Can you work these out from the model? Positions are in its coordinate system, mm. A direction names the side the tool comes from. Coordinates: 2 decimals unless noted, no trailing zeros. Order: outer loops, then holes, each group sorted by start corner. A loop starts at its lowest first (then second) coordinate and runs counter-clockwise, first axis right, second up. Notation, with made-up numbers: (-32.75, 41) -> (1.25, 41) arc R22 cw to (1.25, 71) -> close; hole circle Ø1 at (42.25, -24.75). An arc over 180 degrees is marked (long way). Use a Markdown table: item, result. Add a question column.
1. Suppose I cut it at A-A, the plane z = 0. State how many separate pieces and enclosed holes the cut face has, then the cut area to 3 significant figures.
2. We'd pull the mould along Z, two halves only. Please class faces 5 (the flat face through (-7, 4, 21)), 6 (the flat face through (0, 3, -39.8)), 7 (the flat face through (0, 1, -28)), 8 (the flat face through (0, 12, -4.5)): pulls with the +Z half, pulls with the -Z half, needs draft (parallel to the pull), parting line crosses it, or undercut.
3. If I drill on line 1 along Z through (x, y) = (-7, 3.3); line 2 along X through (y, z) = (3.3, -21.6); line 3 along X through (y, z) = (11.05, 28.8), over which ranges is the centre line in solid material (lowest first)? Write a range as from..to.
4. Suppose I cut it at B-B, the plane y = 5. List the corners of the cut face in (x, z) for me.
5. Suppose I cut it at D-D, the plane y = 27.9. List the corners of the cut face in (x, z) for me, then the cut area to 3 significant figures.
6. For pin 1 Ø7 at (y, z) = (2.5, 27) entering from +X; pin 2 Ø1.2 at (x, y) = (-19.5, 43) entering from -Z; pin 3 Ø3.5 at (x, z) = (-13, 13) entering from -Y; pin 4 Ø8 at (y, z) = (48, 18.5) entering from -X, each with a flat end and sliding along its axis, tell me the tip position at first contact or that it passes through.
7. For faces 1 (the cylindrical face through (-12.01, 1.97, -11.09)), 2 (the flat face through (-19, 43, -8)), 3 (the flat face through (-14, 54.1, 0)), 4 (the flat face through (6.25, 11, -9)), which set-ups out of +Z, -Z, +X, -X, +Y, -Y let a thin tool reach every point of the face, with its end or its side?
8. Suppose I cut it at C-C, the plane z = 13. List the corners of the cut face in (x, y) for me.
```python
from build123d import *

# Parameters (mm, degrees)
SKETCH_1_W                 = 62.3
SKETCH_1_H                 = 34
EXTRUDE_346_DEPTH          = 4
HOLE_WIZARD_M4_1_D         = 4.3
PATTERN_SKETCH_1_OUTLINE_R = 2.15
PATTERN_SKETCH_1_DEPTH     = 4
SKETCH_6_W                 = 22.72
SKETCH_6_H                 = 3
EXTRUDE_2_DEPTH            = 22.8
HOLE_WIZARD_M2_5_1_D       = 2.7
PATTERN_START              = 1
PATTERN_SKETCH_2_OUTLINE_R = 1.35
PATTERN_SKETCH_2_DEPTH     = 3
SKETCH_11_W                = 25.6
SKETCH_11_H                = 4
EXTRUDE_5_DEPTH            = 4
SKETCH_12_W                = 25.6
SKETCH_12_H                = 4
EXTRUDE_6_DEPTH            = 9
SKETCH_13_W                = 25.6
SKETCH_13_H                = 4
EXTRUDE_7_DEPTH            = 16.8
HOLE_WIZARD_M2_1_D         = 2.2
EXTRUDE_START              = -14
EXTRUDE_8_OUTLINE_W        = 12.5
EXTRUDE_8_OUTLINE_H        = 20.251
EXTRUDE_8_OUTLINE_R        = 0.25
EXTRUDE_8_DEPTH            = 9.5
CUT_EXTRUDE_1_REACH        = 67.128
SKETCH_18_R                = 3.2
FILLET_1_RADIUS            = 6.25
FILLET_1_LENGTH            = 9.5
SKETCH_19_W                = 4
SKETCH_19_H                = 24
EXTRUDE_10_DEPTH           = 29
SKETCH_20_W                = 8
SKETCH_20_H                = 1
EXTRUDE_11_DEPTH           = 22.15
CUT_EXTRUDE_3_REACH        = 62.36
SKETCH_22_W                = 1.6
SKETCH_22_H                = 3
FILLET_2_RADIUS            = 0.5
FILLET_2_LENGTH            = 3
FILLET_3_R                 = 0.5
SKETCH_23_W                = 1
SKETCH_23_H                = 9
EXTRUDE_12_DEPTH           = 16.8
HOLE_WIZARD_M3_1_D         = 3.2
EXTRUDE_START_2            = 29
SKETCH_19_2_W              = 4
SKETCH_19_2_H              = 24
EXTRUDE_17_DEPTH           = 29.1
CUT_EXTRUDE_4_REACH        = 90.167
SKETCH_29_W                = 16
SKETCH_29_H                = 21.1
SKETCH_30_W                = 24
SKETCH_30_H                = 8
EXTRUDE_18_DEPTH           = 13.25
CHAMFER_1_SIZE             = 3
FILLET_4_R                 = 2.414214


# Read off the part's stored shape, not the designer's step: 草图阵列1, 草图阵列2, 凸台-拉伸8
with BuildPart() as part:
    # 草图1 → Extrude 346 (new body)
    with BuildSketch(Plane(origin=(0, 0, 0), x_dir=(1, 0, 0), z_dir=(0, 1, 0))):
        Rectangle(SKETCH_1_W, SKETCH_1_H)
    extrude(amount=EXTRUDE_346_DEPTH)

    # M4 间隙孔1 (through all)
    with Locations(Plane(origin=(0, 4, 0), x_dir=(1, 0, 0), z_dir=(0, 1, 0))):
        with Locations((13, -13)):
            Hole(HOLE_WIZARD_M4_1_D / 2)

    # 草图阵列1 outline → 草图阵列1 (cut)
    with BuildSketch(Plane(origin=(0, 0, 0), x_dir=(1, 0, 0), z_dir=(0, 1, 0))):
        with Locations((-13, 13)):
            Circle(PATTERN_SKETCH_1_OUTLINE_R)
        with Locations((-13, -13)):
            Circle(PATTERN_SKETCH_1_OUTLINE_R)
        with Locations((13, 13)):
            Circle(PATTERN_SKETCH_1_OUTLINE_R)
    extrude(amount=PATTERN_SKETCH_1_DEPTH, mode=Mode.SUBTRACT)

    # 草图6 → 凸台-拉伸2 (add)
    with BuildSketch(Plane(origin=(0, 0, -17), x_dir=(-1, 0, 0), z_dir=(0, 0, -1))):
        with Locations((0, 2.5)):
            Rectangle(SKETCH_6_W, SKETCH_6_H)
    extrude(amount=EXTRUDE_2_DEPTH)

    # M2.5 间隙孔1 (through all)
    with Locations(Plane(origin=(0, 4, 0), x_dir=(1, 0, 0), z_dir=(0, 1, 0))):
        with Locations((-7, 35.6)):
            Hole(HOLE_WIZARD_M2_5_1_D / 2)

    # 草图阵列2 outline → 草图阵列2 (cut)
    with BuildSketch(Plane(origin=(0, 0, 0), x_dir=(1, 0, 0), z_dir=(0, 1, 0)).offset(PATTERN_START)):
        with Locations((7, 21.6)):
            Circle(PATTERN_SKETCH_2_OUTLINE_R)
        with Locations((7, 35.6)):
            Circle(PATTERN_SKETCH_2_OUTLINE_R)
        with Locations((-7, 21.6)):
            Circle(PATTERN_SKETCH_2_OUTLINE_R)
    extrude(amount=PATTERN_SKETCH_2_DEPTH, mode=Mode.SUBTRACT)

    # 草图11 → 凸台-拉伸5 (add)
    with BuildSketch(Plane.XY.offset(17)):
        with Locations((0, 2)):
            Rectangle(SKETCH_11_W, SKETCH_11_H)
    extrude(amount=EXTRUDE_5_DEPTH)

    # 草图12 → 凸台-拉伸6 (add)
    with BuildSketch(Plane(origin=(0, 4, 0), x_dir=(1, 0, 0), z_dir=(0, 1, 0))):
        with Locations((0, -19)):
            Rectangle(SKETCH_12_W, SKETCH_12_H)
    extrude(amount=EXTRUDE_6_DEPTH)

    # 草图13 → 凸台-拉伸7 (add)
    with BuildSketch(Plane.XY.offset(21)):
        with Locations((0, 11)):
            Rectangle(SKETCH_13_W, SKETCH_13_H)
    extrude(amount=EXTRUDE_7_DEPTH)

    # M2 间隙孔1 (through all)
    with Locations(Plane(origin=(0, 9, 0), x_dir=(-1, 0, 0), z_dir=(0, -1, 0))):
        with Locations((8.9, -28.8), (-8.9, -28.8)):
            Hole(HOLE_WIZARD_M2_1_D / 2)

    # 凸台-拉伸8 outline → 凸台-拉伸8 (add)
    with BuildSketch(Plane.XY.offset(EXTRUDE_START)):
        with Locations((0, 14.1255)):
            Rectangle(EXTRUDE_8_OUTLINE_W, EXTRUDE_8_OUTLINE_H)
        with Locations((0, 18)):
            Circle(EXTRUDE_8_OUTLINE_R, mode=Mode.SUBTRACT)
    extrude(amount=EXTRUDE_8_DEPTH)

    # 草图18 → 切除-拉伸1 (cut, up to next)
    with BuildSketch(Plane(origin=(0, 0, -14), x_dir=(-1, 0, 0), z_dir=(0, 0, -1)), mode=Mode.PRIVATE) as cut_extrude_1_sk1:
        with Locations((0, 18)):
            Circle(SKETCH_18_R)
    cut_extrude_1_tool1 = extrude(cut_extrude_1_sk1.sketch, amount=-CUT_EXTRUDE_1_REACH, mode=Mode.PRIVATE) & part.part
    add(cut_extrude_1_tool1.solids().sort_by_distance((0, 18, -14))[0], mode=Mode.SUBTRACT)

    # 圆角1: full round fillet: the end face becomes a half cylinder, R = half its width
    fillet_1_face = Plane((0, 24.251, -9.25), x_dir=(0, 0, -1), z_dir=(0, 1, 0))  # on the end face: x along it, z out of the body
    fillet_1_slab = fillet_1_face.offset(-FILLET_1_RADIUS / 2) * Box(FILLET_1_LENGTH, 2 * FILLET_1_RADIUS, FILLET_1_RADIUS, mode=Mode.PRIVATE)  # the body's end, R deep
    fillet_1_round = Plane((0, 18.001, -9.25), x_dir=(0, 1, 0), z_dir=(0, 0, -1)) * Cylinder(FILLET_1_RADIUS, FILLET_1_LENGTH, mode=Mode.PRIVATE)  # its axis R under the face
    add(fillet_1_slab - fillet_1_round, mode=Mode.SUBTRACT)

    # 草图19 → 凸台-拉伸10 (add)
    with BuildSketch(Plane(origin=(0, 4, 0), x_dir=(1, 0, 0), z_dir=(0, 1, 0))):
        with Locations((-19.15, 0)):
            Rectangle(SKETCH_19_W, SKETCH_19_H)
    extrude(amount=EXTRUDE_10_DEPTH)

    # 草图20 → 凸台-拉伸11 (add)
    with BuildSketch(Plane(origin=(-17.15, 0, 0), x_dir=(0, 0, -1), z_dir=(1, 0, 0))):
        with Locations((0, 32.5)):
            Rectangle(SKETCH_20_W, SKETCH_20_H)
    extrude(amount=EXTRUDE_11_DEPTH)

    # 草图22 → 切除-拉伸3 (cut, up to next)
    with BuildSketch(Plane(origin=(0, 33, 0), x_dir=(1, 0, 0), z_dir=(0, 1, 0)), mode=Mode.PRIVATE) as cut_extrude_3_sk1:
        Rectangle(SKETCH_22_W, SKETCH_22_H)
    cut_extrude_3_tool1 = extrude(cut_extrude_3_sk1.sketch, amount=-CUT_EXTRUDE_3_REACH, mode=Mode.PRIVATE) & part.part
    add(cut_extrude_3_tool1.solids().sort_by_distance((0, 33, 0))[0], mode=Mode.SUBTRACT)

    # 圆角2: full round fillet: the end face becomes a half cylinder, R = half its width
    fillet_2_face = Plane((-0.8, 32.5, 0), x_dir=(0, 0, -1), z_dir=(1, 0, 0))  # on the end face: x along it, z out of the body
    fillet_2_slab = fillet_2_face.offset(-FILLET_2_RADIUS / 2) * Box(FILLET_2_LENGTH, 2 * FILLET_2_RADIUS, FILLET_2_RADIUS, mode=Mode.PRIVATE)  # the body's end, R deep
    fillet_2_round = Plane((-1.3, 32.5, 0), x_dir=(1, 0, 0), z_dir=(0, 0, -1)) * Cylinder(FILLET_2_RADIUS, FILLET_2_LENGTH, mode=Mode.PRIVATE)  # its axis R under the face
    add(fillet_2_slab - fillet_2_round, mode=Mode.SUBTRACT)

    # 圆角3
    fillet_3_edges = [part.edges().sort_by_distance(p)[0] for p in [
        (0.8, 33, 0),
    ]]
    fillet(fillet_3_edges, radius=FILLET_3_R)

    # 草图23 → 凸台-拉伸12 (add)
    with BuildSketch(Plane.XY.offset(21)):
        with Locations((0, 4.5)):
            Rectangle(SKETCH_23_W, SKETCH_23_H)
    extrude(amount=EXTRUDE_12_DEPTH)

    # M3 间隙孔1 (through all)
    with Locations(Plane(origin=(-17.15, 0, 0), x_dir=(0, 0, -1), z_dir=(1, 0, 0))):
        with Locations((0, 27.9)):
            Hole(HOLE_WIZARD_M3_1_D / 2)

    # 草图19<2> → 凸台-拉伸17 (add)
    with BuildSketch(Plane(origin=(0, 4, 0), x_dir=(1, 0, 0), z_dir=(0, 1, 0)).offset(EXTRUDE_START_2)):
        with Locations((-19.15, 0)):
            Rectangle(SKETCH_19_2_W, SKETCH_19_2_H)
    extrude(amount=EXTRUDE_17_DEPTH)

    # 草图29 → 切除-拉伸4 (cut, up to next)
    with BuildSketch(Plane(origin=(-17.15, 0, 0), x_dir=(0, 0, -1), z_dir=(1, 0, 0)), mode=Mode.PRIVATE) as cut_extrude_4_sk1:
        with Locations((0, 43.55)):
            Rectangle(SKETCH_29_W, SKETCH_29_H)
    cut_extrude_4_tool1 = extrude(cut_extrude_4_sk1.sketch, amount=-CUT_EXTRUDE_4_REACH, mode=Mode.PRIVATE) & part.part
    add(cut_extrude_4_tool1.solids().sort_by_distance((-17.15, 43.55, 0))[0], mode=Mode.SUBTRACT)

    # 草图30 → 凸台-拉伸18 (add)
    with BuildSketch(Plane(origin=(-17.15, 0, 0), x_dir=(0, 0, -1), z_dir=(1, 0, 0))):
        with Locations((0, 58.1)):
            Rectangle(SKETCH_30_W, SKETCH_30_H)
    extrude(amount=EXTRUDE_18_DEPTH)

    # 倒角1
    chamfer_1_edges = [part.edges().sort_by_distance(p)[0] for p in [
        (-3.9, 62.1, 0),
        (-3.9, 54.1, 0),
    ]]
    chamfer(chamfer_1_edges, length=CHAMFER_1_SIZE)

    # 圆角4
    fillet_4_edges = [part.edges().sort_by_distance(p)[0] for p in [
        (-3.9, 57.1, 0),
        (-3.9, 59.1, 0),
    ]]
    fillet(fillet_4_edges, radius=FILLET_4_R - 0.0001)  # a hair under: the kernel refuses the full size


solid = part.part
```
Worked out:
| question | item | result |
|---|---|---|
| 1 | separate pieces | 4 |
| 1 | enclosed holes | 0 |
| 1 | area | 502 mm² |
| 2 | face 5 | pulls with the +Z half |
| 2 | face 6 | pulls with the -Z half |
| 2 | face 7 | needs draft |
| 2 | face 8 | undercut |
| 3 | line 1 | z = -39.8..-36.95, -34.25..-22.95, -20.25..21 |
| 3 | line 2 | x = -11.36..-8.35, -5.65..5.65, 8.35..11.36 |
| 3 | line 3 | x = -12.8..-10, -7.8..7.8, 10..12.8 |
| 4 | outline | (-21.15, -12) -> (-17.15, -12) -> (-17.15, 12) -> (-21.15, 12) -> close; (-12.8, 17) -> (12.8, 17) -> (12.8, 21) -> (0.5, 21) -> (0.5, 37.8) -> (-0.5, 37.8) -> (-0.5, 21) -> (-12.8, 21) -> close; (-6.25, -14) -> (6.25, -14) -> (6.25, -4.5) -> (-6.25, -4.5) -> close |
| 5 | outline | (-21.15, -12) -> (-17.15, -12) -> (-17.15, -1.6) -> (-21.15, -1.6) -> close; (-21.15, 1.6) -> (-17.15, 1.6) -> (-17.15, 12) -> (-21.15, 12) -> close |
| 5 | area | 83.2 mm² |
| 6 | pin 1 | stops at x = 0.5 |
| 6 | pin 2 | stops at z = -12 |
| 6 | pin 3 | stops at y = 54.1 |
| 6 | pin 4 | passes through |
| 7 | face 1 | -Y |
| 7 | face 2 | +X, -X |
| 7 | face 3 | +X |
| 7 | face 4 | -Z, +X, +Y |
| 8 | outline | (-31.15, 0) -> (-15.15, 0) -> (-15.15, 4) -> (-31.15, 4) -> close; (-10.85, 0) -> (10.85, 0) -> (10.85, 4) -> (-10.85, 4) -> close; (15.15, 0) -> (31.15, 0) -> (31.15, 4) -> (15.15, 4) -> close |
